from build123d import *

# Parameters (mm, degrees)
ESQUISSE2_W             = 110
ESQUISSE2_H             = 30
BOSS_EXTRU_1_DEPTH      = 15
CONG_1_R                = 3
ESQUISSE4_W             = 20
ESQUISSE4_H             = 20
ENL_V_MAT_EXTRU_1_DEPTH = 31
ESQUISSE5_R             = 2.5
ENL_V_MAT_EXTRU_2_DEPTH = 31


with BuildPart() as part:
    # Esquisse2 → Boss.-Extru.1 (new body, symmetric)
    with BuildSketch(Plane(origin=(0, 0, 0), x_dir=(1, 0, 0), z_dir=(0, 1, 0))):
        with Locations((55, 0)):
            Rectangle(ESQUISSE2_W, ESQUISSE2_H)
    extrude(amount=BOSS_EXTRU_1_DEPTH, both=True)

    # Congé1
    cong_1_edges = [part.edges().sort_by_distance(p)[0] for p in [
        (110, 15, 0),
        (0, 15, 0),
        (110, -15, 0),
        (0, -15, 0),
    ]]
    fillet(cong_1_edges, radius=CONG_1_R)

    # Esquisse4 → Enlèv. mat.-Extru.1 (cut, through all)
    with BuildSketch(Plane(origin=(0, 15, 0), x_dir=(1, 0, 0), z_dir=(0, 1, 0))):
        with Locations((100, 0)):
            Rectangle(ESQUISSE4_W, ESQUISSE4_H)
    extrude(amount=-ENL_V_MAT_EXTRU_1_DEPTH, mode=Mode.SUBTRACT)

    # Esquisse5 → Enlèv. mat.-Extru.2 (cut, through all)
    with BuildSketch(Plane(origin=(0, 0, -15), x_dir=(-1, 0, 0), z_dir=(0, 0, -1))):
        with Locations((-105, 10)):
            Circle(ESQUISSE5_R)
        with Locations((-5, 10)):
            Circle(ESQUISSE5_R)
    extrude(amount=-ENL_V_MAT_EXTRU_2_DEPTH, mode=Mode.SUBTRACT)


solid = part.part
Build history of the part. All positions in model axes, mm. A direction names the side the tool comes from. Round coordinates to 2 decimals unless told otherwise and drop trailing zeros. Write each loop counter-clockwise with the first axis right and the second up, starting at its lowest first coordinate (ties: lowest second). Pieces come first, ordered by that corner, then holes. Notation, with made-up numbers: M 46,-39 L 52,-39 A17 ccw 52,-19 Z; hole C 6.5,-24.75 d6. An arc over 180 degrees is marked long. Answer as a JSON object with one key per item and string values. Group by question number.
(1) Mould opens along X. For faces 3 (the cylindrical face through (109.1, 14.14, -12.54)), 4 (the flat face through (54, 0, -15)), 5 (the cylindrical face through (0.86, -14.1, -0.21)), 6 (the cylindrical face through (102.615, 10.751, -12.535)) say: pulls with the +X half, pulls with the -X half, needs draft (parallel to the pull), parting line crosses it, or undercut.
(2) Which spindle directions (+Z, -Z, +X, -X, +Y, -Y) get a long thin tool onto all of the face, cutting with end or side? Do faces 1 (the flat face through (90, 0, 0)), 2 (the cylindrical face through (0.86, 14.1, -0.21)). Say none if no direction does.
(3) Cut at A-A (x = 105). Give the cut face in (y, z).
(4) Cut at C-C (y = 10). Give the cut face in (x, z), and give its area (3 significant figures).
(5) Drill centre lines: L1, parallel to Y at x = 105, z = -11.15; L2, parallel to Z at x = 98, y = 11.75; L3, parallel to X at y = 6, z = -2.75. Where is each one in solid material? Low to high.
(6) Flat gauge pin, fed straight in: pin 1 (2 mm diameter, centred on y = -8.5, z = -3.5, fed in from +X). Where does the tip first touch, or does it go through?
(7) Cut at B-B (z = 4.75). Give the cut face in (x, y), and give its area (3 significant figures).
(8) Cut at D-D (x = 5). Give the cut face in (y, z).
Responses:
{
 "1": {"face 3": "pulls with the +X half", "face 4": "needs draft", "face 5": "pulls with the -X half", "face 6": "undercut"},
 "2": {"face 1": "+X, +Y, -Y", "face 2": "+Z, -Z, -X, +Y"},
 "3": {"outline": "M -15,-15 L 7.5,-15 L 7.5,-10 L -15,-10 Z; M -15,10 L 7.5,10 L 7.5,15 L -15,15 Z; M 12.5,-15 L 15,-15 L 15,-10 L 12.5,-10 Z; M 12.5,10 L 15,10 L 15,15 L 12.5,15 Z"},
 "4": {"outline": "M 0,-15 L 2.5,-15 L 2.5,15 L 0,15 Z; M 7.5,-15 L 102.5,-15 L 102.5,-10 L 90,-10 L 90,10 L 102.5,10 L 102.5,15 L 7.5,15 Z; M 107.5,-15 L 110,-15 L 110,-10 L 107.5,-10 Z; M 107.5,10 L 110,10 L 110,15 L 107.5,15 Z", "area": "2,700 mm2"},
 "5": {"L1": "y = -15 to 7.5, 12.5 to 15", "L2": "z = -15 to -10, 10 to 15", "L3": "x = 0 to 90"},
 "6": {"pin 1": "stops at x = 90"},
 "7": {"outline": "M 0,-12 A3 ccw 3,-15 L 90,-15 L 90,15 L 3,15 A3 ccw 0,12 Z; hole C 5,10 d5", "area": "2,680 mm2"},
 "8": {"outline": "M -15,-15 L 7.5,-15 L 7.5,15 L -15,15 Z; M 12.5,-15 L 15,-15 L 15,15 L 12.5,15 Z"}
}
